```python
from build123d import *

# Parameters (mm, degrees)
F0_W     = 7.5
F0_H     = 10.5
F1_DEPTH = 10.5
F2_SIZE2 = 3
F2_SIZE  = 1.5
F3_SIZE2 = 1
F3_SIZE  = 3
F4_R     = 1.5
F5_DEPTH = 2
F6_W     = 4
F6_H     = 5
F7_DEPTH = 0.5


with BuildPart() as f1:
    # F0 (on Front) → F1 (new body)
    with BuildSketch(Plane.XZ):
        with Locations((-3.75, 5.25)):
            Rectangle(F0_W, F0_H)
    extrude(amount=-F1_DEPTH)

    # F2
    f2_edges = [f1.edges().sort_by_distance(p)[0] for p in [
        (-7.5, 5.25, 10.5),
    ]]
    f2_side = f1.faces().sort_by_distance((-3.75, 5.25, 10.5))[0]
    chamfer(f2_edges, length=F2_SIZE, length2=F2_SIZE2, reference=f2_side)

    # F3
    f3_edges = [f1.edges().sort_by_distance(p)[0] for p in [
        (0, 5.25, 10.5),
    ]]
    f3_side = f1.faces().sort_by_distance((0, 5.25, 5.25))[0]
    chamfer(f3_edges, length=F3_SIZE, length2=F3_SIZE2, reference=f3_side)

    # F4 (on face) → F5 (cut)
    with BuildSketch(Plane.XY.offset(10.5)):
        with Locations((-3.5, 2.75)):
            Circle(F4_R)
        with Locations((-3.5, 7.75)):
            Circle(F4_R)
    extrude(amount=-F5_DEPTH, mode=Mode.SUBTRACT)

    # F6 (on face) → F7 (cut)
    with BuildSketch(Plane.YZ):
        with Locations((2.75, 3)):
            Rectangle(F6_W, F6_H)
        with Locations((7.75, 3)):
            Rectangle(F6_W, F6_H)
    extrude(amount=-F7_DEPTH, mode=Mode.SUBTRACT)


solid = f1.part
```
Could you check a few things on this model? Use its own coordinates, in mm. A direction names the side the tool comes from. Give positions to 0.01 mm unless a question says otherwise; leave off trailing zeros. Write each loop counter-clockwise with the first axis right and the second up, starting at its lowest first coordinate (ties: lowest second). Pieces come first, ordered by that corner, then holes. Notation, with made-up numbers: (-13.75, 82) - (-8.75, 82) arc R18 cw to (-8.75, 102) - close; hole circle Ø8 at (-18, 22). An arc over 180 degrees is marked (long way). One line per item, written item: value. Start each with the question number.
Item 1: I'm going to push flat-ended pins straight in: pin 1 (1.2 mm diameter, centred on y = 2, z = 2, fed in from +X); pin 2 (1.5 mm diameter, centred on x = -3, y = 2.5, fed in from +Z). Where does each tip first touch, or does it pass through?
Item 2: Imagine slicing it at C-C, the plane z = 4.75. List the corners of the cut face in (x, y) for me, and give its area (4 significant figures).
Item 3: Imagine slicing it at B-B, the plane x = -3.5. List the corners of the cut face in (y, z) for me, and give its area (4 significant figures).
Item 4: Which directions (+Z, -Z, +X, -X, +Y, -Y) give clear straight access to the entire face, cutting with the end or side of a thin tool? Please do faces 5 (the face through (0, 5, 4)), 6 (the face through (-0.5, 3, 3)), 7 (the face through (-4, 3, 8.5)).
Item 5: Please list where these lines run through material, in increasing order: line 1 (Y direction, x = -3.5, z = 9.6); line 2 (X direction, y = 2.5, z = 9); line 3 (Z direction, x = -6.5, y = 5.5). Write a range as from..to.
Item 6: If we mould it in two halves opening along Y, with no side actions, what happens to faces 1 (the face through (-4, 8, 8.5)), 2 (the face through (-7.5, 5, 4)), 3 (the face through (-4, 10.5, 5)), 4 (the face through (-4, 0, 5))? For each: +Y half, -Y half, draft (parallel to the pull), parting line (faces both ways), or undercut.
Item 7: Imagine slicing it at D-D, the plane y = 7.75. List the corners of the cut face in (x, z) for me, and give its area (3 significant figures).
Item 8: Imagine slicing it at A-A, the plane y = 9.5. List the corners of the cut face in (x, z) for me.
Geometry says:
1. pin 1: x = -0.5
1. pin 2: z = 8.5
2. outline: (-7.5, 0) - (0, 0) - (0, 0.75) - (-0.5, 0.75) - (-0.5, 4.75) - (0, 4.75) - (0, 5.75) - (-0.5, 5.75) - (-0.5, 9.75) - (0, 9.75) - (0, 10.5) - (-7.5, 10.5) - close
2. area: 74.75 mm^2
3. outline: (0, 0) - (10.5, 0) - (10.5, 10.5) - (9.25, 10.5) - (9.25, 8.5) - (6.25, 8.5) - (6.25, 10.5) - (4.25, 10.5) - (4.25, 8.5) - (1.25, 8.5) - (1.25, 10.5) - (0, 10.5) - close
3. area: 98.25 mm^2
4. face 5: +Z, -Z, +X, +Y, -Y
4. face 6: +X
4. face 7: +Z
5. line 1: 0..1.25, 4.25..6.25, 9.25..10.5
5. line 2: -6.75..-4.98, -2.02..-0.5
5. line 3: 0..9.5
6. face 1: undercut
6. face 2: draft
6. face 3: +Y half
6. face 4: -Y half
7. outline: (-7.5, 0) - (0, 0) - (0, 0.5) - (-0.5, 0.5) - (-0.5, 5.5) - (0, 5.5) - (0, 7.5) - (-1, 10.5) - (-2, 10.5) - (-2, 8.5) - (-5, 8.5) - (-5, 10.5) - (-6, 10.5) - (-7.5, 7.5) - close
7. area: 66.5 mm^2
8. outline: (-7.5, 0) - (0, 0) - (0, 0.5) - (-0.5, 0.5) - (-0.5, 5.5) - (0, 5.5) - (0, 7.5) - (-1, 10.5) - (-6, 10.5) - (-7.5, 7.5) - close
